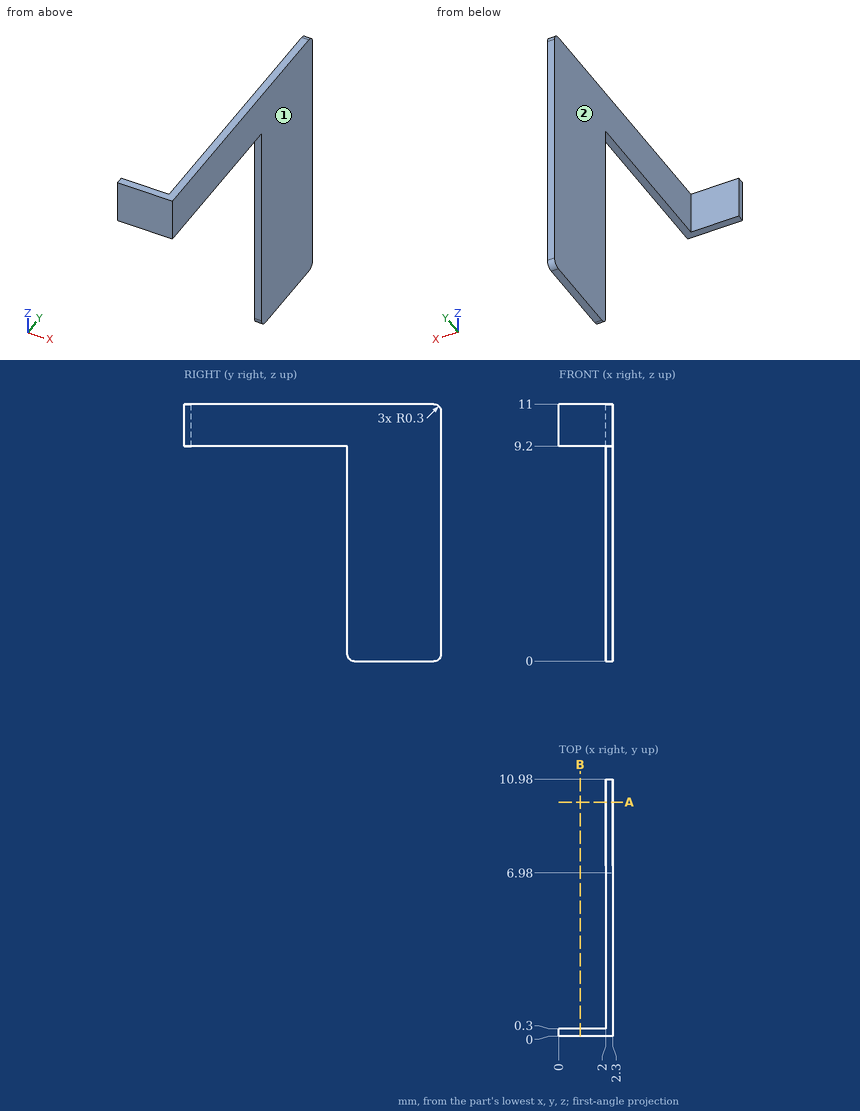
For this review, use the dimensioned drawing (mm, ordinates from the lowest corner) and the shaded views. A direction names the side the tool comes from. Round coordinates to 2 decimals unless told otherwise and drop trailing zeros. Order: outer loops, then holes, each group sorted by start corner. A loop starts at its lowest first (then second) coordinate and runs counter-clockwise, first axis right, second up. Notation, with made-up numbers: M 61,37.25 L 117,37.25 A13 ccw 117,48.25 Z; hole C 51.5,33.5 d7. An arc over 180 degrees is marked long. Use a Markdown table: item, result.
1) Consider section A-A (y = 10). Write out the cut boundary in (x, z).
Report:
| item | result |
|---|---|
| outline | M 2,0 L 2.3,0 L 2.3,11 L 2,11 Z |
2) Wall thickness on line 1 along X through (y, z) = (10.5, 3); line 2 along Z through (x, y) = (2.2, 3): over which ranges is each line inside the solid? List them lowest first. Write a range as [from, to].
Report:
| item | result |
|---|---|
| line 1 | [2, 2.3] |
| line 2 | [9.2, 11] |
3) Consider section B-B (x = 0.9). Write out the cut boundary in (y, z), then the cut area to 3 significant figures.
Report:
| item | result |
|---|---|
| outline | M 0,9.2 L 0.3,9.2 L 0.3,11 L 0,11 Z |
| area | 0.540 mm^2 |
4) Insertion check: pin 1 (5.5 mm diameter, centred on y = 7.5, z = 4.5, fed in from -X). The pin has a flat end and moves straight along its axis. Give the tip position at first contact, or say it passes through.
Report:
| item | result |
|---|---|
| pin 1 | x = 2 |
5) Tool access review of the marked faces 1 and 2: name each direction out of +Z, -Z, +X, -X, +Y, -Y from which nothing blocks a thin tool from reaching the whole face with its end or side.
Report:
| item | result |
|---|---|
| face 1 | +Z, -Z, +X, +Y, -Y |
| face 2 | +Z, -Z, -X, +Y |
